Verification items for the finished model (mm, model axes). A direction names the side the tool comes from. Round coordinates to 2 decimals unless told otherwise and drop trailing zeros. Write each loop counter-clockwise with the first axis right and the second up, starting at its lowest first coordinate (ties: lowest second). Pieces come first, ordered by that corner, then holes. Notation, with made-up numbers: (83.25, 9) - (122.25, 9) arc R30 ccw to (122.25, 46) - close; hole circle Ø5 at (27, 52.25). An arc over 180 degrees is marked (long way). Answer as a JSON object with one key per item and string values.
```python
from build123d import *

# Parameters (mm, degrees)
ESQUISSE1_W             = 43.6
ESQUISSE1_H             = 43.6
BOSS_EXTRU_1_DEPTH      = 6
CONG_1_R                = 10
ESQUISSE2_R             = 1.5
ESQUISSE2_W             = 15.6
ESQUISSE2_H             = 6
ENL_V_MAT_EXTRU_1_DEPTH = 6
ESQUISSE3_R             = 2.995
ENL_V_MAT_EXTRU_2_DEPTH = 3


with BuildPart() as part:
    # Esquisse1 → Boss.-Extru.1 (new body)
    with BuildSketch(Plane.XY):
        with Locations((21.8, 21.8)):
            Rectangle(ESQUISSE1_W, ESQUISSE1_H)
    extrude(amount=BOSS_EXTRU_1_DEPTH)

    # Congé1
    cong_1_edges = [part.edges().sort_by_distance(p)[0] for p in [
        (0, 43.6, 3),
        (43.6, 43.6, 3),
        (43.6, 0, 3),
        (0, 0, 3),
    ]]
    fillet(cong_1_edges, radius=CONG_1_R)

    # Esquisse2 → Enlèv. mat.-Extru.1 (cut)
    with BuildSketch(Plane.XY.offset(6)):
        with Locations((8, 21.8)):
            Circle(ESQUISSE2_R)
        with Locations((35.6, 21.8)):
            Circle(ESQUISSE2_R)
        with Locations((21.8, 21.8)):
            Rectangle(ESQUISSE2_W, ESQUISSE2_H)
    extrude(amount=-ENL_V_MAT_EXTRU_1_DEPTH, mode=Mode.SUBTRACT)

    # Esquisse3 → Enlèv. mat.-Extru.2 (cut)
    with BuildSketch(Plane.XY.offset(6)):
        with Locations((8, 21.8)):
            Circle(ESQUISSE3_R)
        with Locations((35.6, 21.8)):
            Circle(ESQUISSE3_R)
    extrude(amount=-ENL_V_MAT_EXTRU_2_DEPTH, mode=Mode.SUBTRACT)


solid = part.part
```
Q1. Gauge pin test, flat ends, axial feed: P1, Ø8, axis at x = 17.5, y = 5.5, coming from the -Z side; P2, Ø1, axis at x = 38.5, z = 3.5, coming from the -Y side; P3, Ø2.5, axis at x = 35.6, y = 21.8, coming from the -Z side; P4, Ø2, axis at y = 35, z = 2, coming from the -X side. Record the tip position at first contact, or that the pin passes through.
Geometry check:
{"P1": "stops at z = 0", "P2": "stops at y = 1.02", "P3": "passes through", "P4": "stops at x = 0.01"}
Q2. Section check C-C, the plane z = 2.4. Record the cut outline in (x, y).
Geometry check:
{"outline": "(0, 10) arc R10 ccw to (10, 0) - (33.6, 0) arc R10 ccw to (43.6, 10) - (43.6, 33.6) arc R10 ccw to (33.6, 43.6) - (10, 43.6) arc R10 ccw to (0, 33.6) - close; hole circle Ø3 at (8, 21.8); hole (14, 18.8) - (29.6, 18.8) - (29.6, 24.8) - (14, 24.8) - close; hole circle Ø3 at (35.6, 21.8)"}
Q3. Material ranges on line 1 along Y through (x, z) = (29.5, 3.7); line 2 along X through (y, z) = (21.5, 1.4); line 3 along Y through (x, z) = (8, 0.85), recorded low to high. Write a range as [from, to].
Geometry check:
{"line 1": "y = [0, 18.8], [24.8, 43.6]", "line 2": "x = [0, 6.53], [9.47, 14], [29.6, 34.13], [37.07, 43.6]", "line 3": "y = [0.2, 20.3], [23.3, 43.4]"}
Q4. Section check A-A, the plane x = 18. Record the cut outline in (y, z), then the cut area to 3 significant figures.
Geometry check:
{"outline": "(0, 0) - (18.8, 0) - (18.8, 6) - (0, 6) - close; (24.8, 0) - (43.6, 0) - (43.6, 6) - (24.8, 6) - close", "area": "226 mm2"}
Q5. Set-up check for faces 4 (the flat face through (22, 0, 3)), 5 (the flat face through (9.3, 20.5, 3)), 6 (the flat face through (22, 24.8, 3)): record each of +Z, -Z, +X, -X, +Y, -Y from which the full face is reachable in a straight line by a thin tool's end or side.
Geometry check:
{"face 4": "+Z, -Z, +X, -X, -Y", "face 5": "+Z", "face 6": "+Z, -Z"}
Q6. Section check D-D, the plane z = 5.05. Record the cut outline in (x, y) (3 decimals).
Geometry check:
{"outline": "(0, 10) arc R10 ccw to (10, 0) - (33.6, 0) arc R10 ccw to (43.6, 10) - (43.6, 33.6) arc R10 ccw to (33.6, 43.6) - (10, 43.6) arc R10 ccw to (0, 33.6) - close; hole circle Ø5.99 at (8, 21.8); hole (14, 18.8) - (29.6, 18.8) - (29.6, 24.8) - (14, 24.8) - close; hole circle Ø5.99 at (35.6, 21.8)"}
Q7. Release check for a two-part mould opening along X. For faces 1 (the cylindrical face through (40.75, 40.59, 3.04)), 2 (the cylindrical face through (2.85, 3.01, 3.04)), 3 (the cylindrical face through (33.39, 23.82, 4.52)) record: released by +X, released by -X, zero draft, split by the parting line, or undercut.
Geometry check:
{"face 1": "released by +X", "face 2": "released by -X", "face 3": "undercut"}
Q8. Section check B-B, the plane y = 21.8. Record the cut outline in (x, z) (3 decimals).
Geometry check:
{"outline": "(0, 0) - (6.5, 0) - (6.5, 3) - (5.005, 3) - (5.005, 6) - (0, 6) - close; (9.5, 0) - (14, 0) - (14, 6) - (10.995, 6) - (10.995, 3) - (9.5, 3) - close; (29.6, 0) - (34.1, 0) - (34.1, 3) - (32.605, 3) - (32.605, 6) - (29.6, 6) - close; (37.1, 0) - (43.6, 0) - (43.6, 6) - (38.595, 6) - (38.595, 3) - (37.1, 3) - close"}
